Drawing for the job (mm, zero at the part's lowest x, y, z). Round coordinates to 2 decimals unless told otherwise and drop trailing zeros. Write each loop counter-clockwise with the first axis right and the second up, starting at its lowest first coordinate (ties: lowest second). Pieces come first, ordered by that corner, then holes. Notation, with made-up numbers: (54, -0.75) -> (81, -0.75) arc R19 ccw to (81, 4.25) -> close; hole circle Ø11 at (-26.75, -39.5). An arc over 180 degrees is marked (long way). Answer in a Markdown table with one row per item. Add a question column.
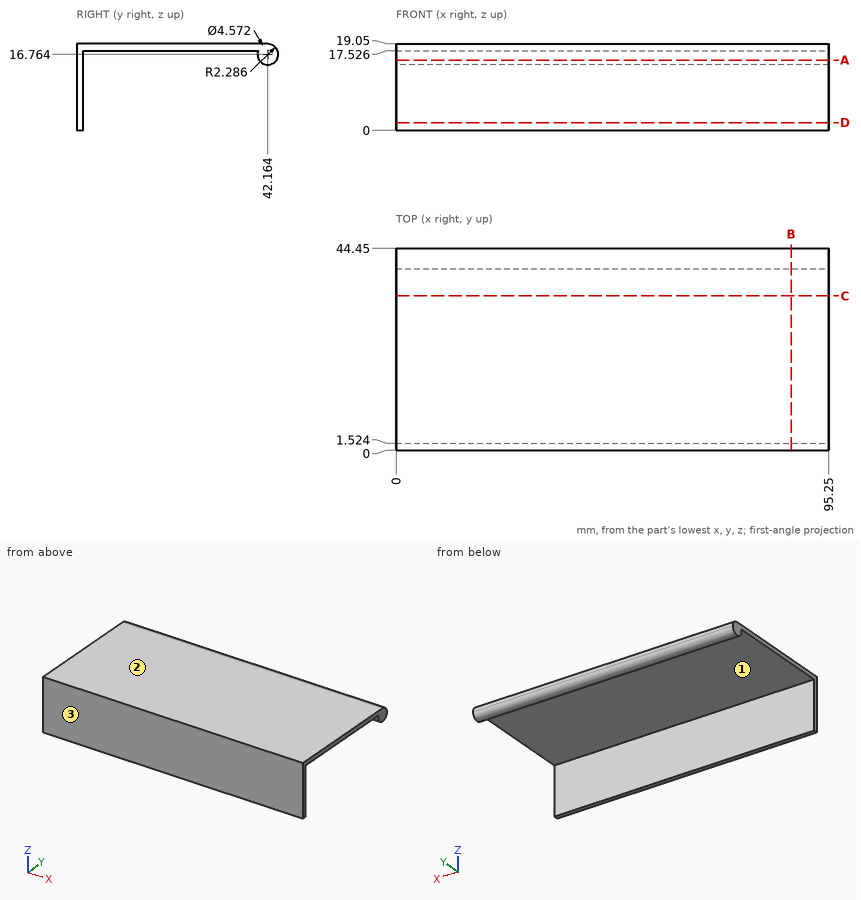
(1) Probe line 1 along Y through (x, z) = (7, 12.5); line 2 along Z through (x, y) = (17, 20.5); line 3 along Y through (x, z) = (10.5, 15.75). List the from-to ranges inside material, lowest first.
(2) Drop a flat-ended pin along its axis: P1, Ø11.5, axis at x = 66, y = 21, coming from the -Z side. Give the stop position or say it passes through.
(3) Saw through at C-C (y = 34). List the corners of the cut face in (x, z), plus the area to 3 significant figures.
(4) Mould opens along Y. For the marked faces 1, 2 and 3 say: pulls with the +Y half, pulls with the -Y half, needs draft (parallel to the pull), parting line crosses it, or undercut.
(5) Saw through at A-A (z = 15.5). List the corners of the cut face in (x, y).
(6) Saw through at D-D (z = 1.75). List the corners of the cut face in (x, y).
(7) Saw through at B-B (x = 87). List the corners of the cut face in (y, z), plus the area to 3 significant figures.
Answer sheet:
| question | item | result |
|---|---|---|
| 1 | line 1 | y = 0 to 1.52 |
| 1 | line 2 | z = 17.53 to 19.05 |
| 1 | line 3 | y = 0 to 1.52, 40.12 to 44.21 |
| 2 | P1 | stops at z = 17.53 |
| 3 | outline | (0, 17.53) -> (95.25, 17.53) -> (95.25, 19.05) -> (0, 19.05) -> close |
| 3 | area | 145 mm² |
| 4 | face 1 | undercut |
| 4 | face 2 | needs draft |
| 4 | face 3 | pulls with the -Y half |
| 5 | outline | (0, 0) -> (95.25, 0) -> (95.25, 1.52) -> (0, 1.52) -> close; (0, 40.26) -> (95.25, 40.26) -> (95.25, 44.07) -> (0, 44.07) -> close |
| 6 | outline | (0, 0) -> (95.25, 0) -> (95.25, 1.52) -> (0, 1.52) -> close |
| 7 | outline | (0, 0) -> (1.52, 0) -> (1.52, 17.53) -> (40.01, 17.53) arc R2.29 ccw (long way) to (42.16, 19.05) -> (0, 19.05) -> close |
| 7 | area | 105 mm² |
